Geometry check sheet. Reference: drawing and pictorial views, mm from the part's lowest x, y, z. A direction names the side the tool comes from. Round coordinates to 2 decimals unless told otherwise and drop trailing zeros. Order: outer loops, then holes, each group sorted by start corner. A loop starts at its lowest first (then second) coordinate and runs counter-clockwise, first axis right, second up.
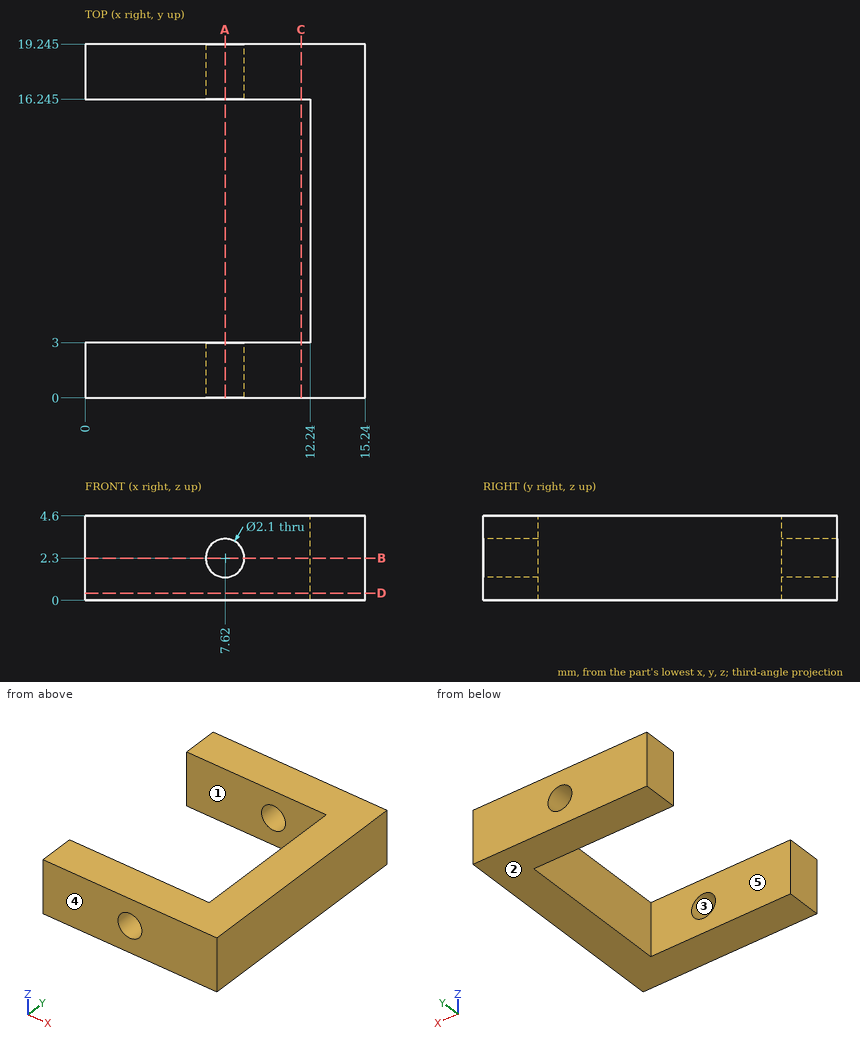
1) Tool access check on the marked faces 1 and 2. Record the directions out of +Z, -Z, +X, -X, +Y, -Y that give a thin tool (end or side, any length) a straight path to the whole face; none if there is none.
2) Sectioned sample at C-C on x = 11.75. Record the cut outline in (y, z) (3 decimals), then the cut area to 3 significant figures.
3) Draft check along Y on the marked faces 3, 4 and 5. Enter one of: released by +Y, released by -Y, zero draft, split by the parting line, or undercut.
4) Go/stop test with a flat-tipped pin: pin 1 Ø1.9 at (x, z) = (7.62, 2.3) entering from +Y. Record where the tip stops, or that it passes through.
5) Sectioned sample at A-A on x = 7.62. Record the cut outline in (y, z) (3 decimals).
6) Sectioned sample at B-B on z = 2.3. Record the cut outline in (x, y) (3 decimals).
7) Scan lines: probe 1 along Y at (x, z) = (11.5, 2.2) (3 decimals); probe 2 along Z at (x, y) = (7.62, 16.95); probe 3 along X at (y, z) = (13.75, 2.2). Record each from-to range of solid material in increasing order.
8) Sectioned sample at D-D on z = 0.4. Record the cut outline in (x, y) (3 decimals), then the cut area to 3 significant figures.
Returned:
1. face 1: +Z, -Z, -X
1. face 2: -Z, +X, -X, +Y, -Y
2. outline: (0, 0) - (3, 0) - (3, 4.6) - (0, 4.6) - close; (16.245, 0) - (19.245, 0) - (19.245, 4.6) - (16.245, 4.6) - close
2. area: 27.6 mm2
3. face 3: zero draft
3. face 4: released by -Y
3. face 5: undercut
4. pin 1: passes through
5. outline: (0, 0) - (3, 0) - (3, 1.25) - (0, 1.25) - close; (0, 3.35) - (3, 3.35) - (3, 4.6) - (0, 4.6) - close; (16.245, 0) - (19.245, 0) - (19.245, 1.25) - (16.245, 1.25) - close; (16.245, 3.35) - (19.245, 3.35) - (19.245, 4.6) - (16.245, 4.6) - close
6. outline: (0, 0) - (6.57, 0) - (6.57, 3) - (0, 3) - close; (0, 16.245) - (6.57, 16.245) - (6.57, 19.245) - (0, 19.245) - close; (8.67, 0) - (15.24, 0) - (15.24, 19.245) - (8.67, 19.245) - (8.67, 16.245) - (12.24, 16.245) - (12.24, 3) - (8.67, 3) - close
7. probe 1: y = 0 to 3, 16.245 to 19.245
7. probe 2: z = 0 to 1.25, 3.35 to 4.6
7. probe 3: x = 12.24 to 15.24
8. outline: (0, 0) - (15.24, 0) - (15.24, 19.245) - (0, 19.245) - (0, 16.245) - (12.24, 16.245) - (12.24, 3) - (0, 3) - close
8. area: 131 mm2
